Check sheet for the modelled part. Datum: model origin and axes. Units: mm. A direction names the side the tool comes from. Round coordinates to 2 decimals unless told otherwise and drop trailing zeros. Loops run counter-clockwise (first coordinate to the right, second up) from the corner with the lowest first, then second, coordinate; pieces in that order, holes last. Notation, with made-up numbers: (-32, 17.25) -> (7, 17.25) arc R25 cw to (7, 54.25) -> close; hole circle Ø1 at (75, 31.5). An arc over 180 degrees is marked (long way). One line per item, written item: value. Start each with the question number.
1. Cross-section at C-C on x = 89.5. Record the cut outline in (y, z), then the cut area to 3 significant figures.
2. Set-up check for faces 1 (the face through (29, 62, -7)), 2 (the face through (112, -60, -6)), 3 (the face through (33, 66, -7)), 4 (the face through (115, 62, -7)), 5 (the face through (-61.6, -51.1, 2.5)): record each of +Z, -Z, +X, -X, +Y, -Y from which the full face is reachable in a straight line by a thin tool's end or side.
3. Release check for a two-part mould opening along Y. For faces 6 (the face through (109, -63, -6)), 7 (the face through (31, 2, 5)), 8 (the face through (32.14, 84.86, 2.54)), 9 (the face through (127.15, -101.99, 2.46)) record: +Y half, -Y half, draft (parallel to the pull), parting line (faces both ways), or undercut.
4. Cross-section at B-B on y = 4.5. Record the cut outline in (x, z).
5. Cross-section at A-A on z = -12. Record the cut outline in (x, y).
6. Go/stop test with flat-tipped pins: pin 1 (3 mm diameter, centred on x = 49.5, y = 63.5, fed in from +Z); pin 2 (4 mm diameter, centred on x = 34.5, z = -7, fed in from +Y); pin 3 (1.5 mm diameter, centred on x = -101.5, z = 2.5, fed in from +Y); pin 4 (3.5 mm diameter, centred on x = -16.85, y = 58.25, fed in from -Z). Record where each tip stops, or that it passes through.
7. Material ranges on L1, parallel to Y at x = 79.5, z = 3.75; L2, parallel to X at y = 58.25, z = 2.45; L3, parallel to Y at x = -34.85, z = 2, recorded low to high.
from build123d import *

# Parameters (mm, degrees)
EXTRUDE_1_DEPTH       = 5
CUT_EXTRUDE_1_DEPTH   = 185.623942109
CUT_EXTRUDE_2_DEPTH   = 185.623942109
EXTRUDE_2_DEPTH       = 15
CUT_EXTRUDE_3_DEPTH   = 10
CUT_EXTRUDE_4_DEPTH   = 10
MIRROR_2_COPY_1_DEPTH = 15
MIRROR_2_COPY_2_DEPTH = 10
MIRROR_2_COPY_3_DEPTH = 10
SKETCH_7_R            = 1.6
CUT_EXTRUDE_5_DEPTH   = 186.16479147
SKETCH_8_R            = 1.6
CUT_EXTRUDE_6_DEPTH   = 186.16479147


with BuildPart() as part:
    # 草图1 → 凸台-拉伸1 (new body)
    with BuildSketch(Plane.XY):
        with BuildLine():
            Line((-51, 115), (-51, 121))
            ThreePointArc((-51, 121), (-48.071067812, 128.071067812), (-41, 131))
            Line((-41, 131), (29, 131))
            ThreePointArc((29, 131), (36.071067812, 128.071067812), (39, 121))
            Line((39, 121), (39, 115))
            ThreePointArc((39, 115), (41.928932188, 107.928932188), (49, 105))
            Line((49, 105), (120, 105))
            ThreePointArc((120, 105), (127.071067812, 102.071067812), (130, 95))
            Line((130, 95), (130, -95))
            ThreePointArc((130, -95), (127.071067812, -102.071067812), (120, -105))
            Line((120, -105), (49, -105))
            ThreePointArc((49, -105), (41.928932188, -107.928932188), (39, -115))
            Line((39, -115), (39, -121))
            ThreePointArc((39, -121), (36.071067812, -128.071067812), (29, -131))
            Line((29, -131), (-41, -131))
            ThreePointArc((-41, -131), (-48.071067812, -128.071067812), (-51, -121))
            Line((-51, -121), (-51, -115))
            ThreePointArc((-51, -115), (-53.928932188, -107.928932188), (-61, -105))
            Line((-61, -105), (-120, -105))
            ThreePointArc((-120, -105), (-127.071067812, -102.071067812), (-130, -95))
            Line((-130, -95), (-130, 95))
            ThreePointArc((-130, 95), (-127.071067812, 102.071067812), (-120, 105))
            Line((-120, 105), (-61, 105))
            ThreePointArc((-61, 105), (-53.928932188, 107.928932188), (-51, 115))
        make_face()
    extrude(amount=EXTRUDE_1_DEPTH)

    # 草图2 → 切除-拉伸1 (cut, through all)
    with BuildSketch(Plane.XY.offset(5)):
        with BuildLine():
            Line((10.846153846, -93.730769231), (52.846153846, -76.230769231))
            ThreePointArc((52.846153846, -76.230769231), (55.664100589, -76.503849117), (57, -79))
            Line((57, -79), (57, -96.5))
            ThreePointArc((57, -96.5), (56.121320344, -98.621320344), (54, -99.5))
            Line((54, -99.5), (12, -99.5))
            ThreePointArc((12, -99.5), (9.058257973, -97.088348405), (10.846153846, -93.730769231))
        make_face()
        Polygon((-108, 99.5), (-86, 99.5), (-82, 95.5), (-82, 73.5), (-86, 69.5), (-108, 69.5), (-112, 73.5), (-112, 95.5), align=None)
        Polygon((-108, -67), (-86, -67), (-82, -71), (-82, -93), (-86, -97), (-108, -97), (-112, -93), (-112, -71), align=None)
        Polygon((86, 97), (108, 97), (112, 93), (112, 76), (108, 72), (86, 72), (82, 76), (82, 93), align=None)
        Polygon((86, -69.5), (108, -69.5), (112, -73.5), (112, -90.5), (108, -94.5), (86, -94.5), (82, -90.5), (82, -73.5), align=None)
        with BuildLine():
            Line((12, 99.5), (54, 99.5))
            ThreePointArc((54, 99.5), (56.121320344, 98.621320344), (57, 96.5))
            Line((57, 96.5), (57, 79))
            ThreePointArc((57, 79), (55.664100589, 76.503849117), (52.846153846, 76.230769231))
            Line((52.846153846, 76.230769231), (10.846153846, 93.730769231))
            ThreePointArc((10.846153846, 93.730769231), (9.058257973, 97.088348405), (12, 99.5))
        make_face()
    extrude(amount=-CUT_EXTRUDE_1_DEPTH, mode=Mode.SUBTRACT)

    # 草图3 → 切除-拉伸2 (cut, through all)
    with BuildSketch(Plane(origin=(0, 0, 0), x_dir=(-1, 0, 0), z_dir=(0, 0, -1))):
        Polygon((57.7, 55), (-18, 55), (-26, 47), (-26, -47), (-18, -55), (57.7, -55), (65.7, -47), (65.7, 47), align=None)
    extrude(amount=-CUT_EXTRUDE_2_DEPTH, mode=Mode.SUBTRACT)

    # 草图4 → 凸台-拉伸2 (add)
    with BuildSketch(Plane(origin=(0, 0, 0), x_dir=(-1, 0, 0), z_dir=(0, 0, -1))):
        Polygon((-29, -55), (-29, -66), (-40, -66), (-40, -63), (-32, -63), (-32, -55), align=None)
    extrude_2 = extrude(amount=EXTRUDE_2_DEPTH)

    # 草图5 → 切除-拉伸3 (cut)
    with BuildSketch(Plane.XZ.offset(66)):
        Polygon((40, -5), (34.5, -15), (40, -15), align=None)
    cut_extrude_3 = extrude(amount=-CUT_EXTRUDE_3_DEPTH, mode=Mode.SUBTRACT)

    # 草图6 → 切除-拉伸4 (cut)
    with BuildSketch(Plane.ZY.offset(-29)):
        Polygon((-15, -60.5), (-5, -55), (-15, -55), align=None)
    cut_extrude_4 = extrude(amount=-CUT_EXTRUDE_4_DEPTH, mode=Mode.SUBTRACT)

    # 镜向1: 凸台-拉伸2, 切除-拉伸3, 切除-拉伸4 across plane
    add(extrude_2.mirror(Plane.ZY.offset(-72)))
    add(cut_extrude_3.mirror(Plane.ZY.offset(-72)), mode=Mode.SUBTRACT)
    add(cut_extrude_4.mirror(Plane.ZY.offset(-72)), mode=Mode.SUBTRACT)

    # 镜向2: 凸台-拉伸2, 切除-拉伸3, 切除-拉伸4 across plane
    add(extrude_2.mirror(Plane.ZX))
    add(cut_extrude_3.mirror(Plane.ZX), mode=Mode.SUBTRACT)
    add(cut_extrude_4.mirror(Plane.ZX), mode=Mode.SUBTRACT)

    # 镜向2 copy 1 sketch → 镜向2 copy 1 (add)
    with BuildSketch(Plane(origin=(144, 0, 0), x_dir=(1, 0, 0), z_dir=(0, 0, -1))):
        Polygon((-29, -55), (-29, -66), (-40, -66), (-40, -63), (-32, -63), (-32, -55), align=None)
    extrude(amount=MIRROR_2_COPY_1_DEPTH)

    # 镜向2 copy 2 sketch → 镜向2 copy 2 (cut)
    with BuildSketch(Plane(origin=(144, 66, 0), x_dir=(-1, 0, 0), z_dir=(0, 1, 0))):
        Polygon((40, -5), (34.5, -15), (40, -15), align=None)
    extrude(amount=-MIRROR_2_COPY_2_DEPTH, mode=Mode.SUBTRACT)

    # 镜向2 copy 3 sketch → 镜向2 copy 3 (cut)
    with BuildSketch(Plane(origin=(115, 0, 0), x_dir=(0, 0, 1), z_dir=(1, 0, 0))):
        Polygon((-15, -60.5), (-5, -55), (-15, -55), align=None)
    extrude(amount=-MIRROR_2_COPY_3_DEPTH, mode=Mode.SUBTRACT)

    # 草图7 → 切除-拉伸5 (cut, through all)
    with BuildSketch(Plane(origin=(0, 0, 0), x_dir=(-1, 0, 0), z_dir=(0, 0, -1))):
        with Locations((16.85, -58.25)):
            Circle(SKETCH_7_R)
        with Locations((22.85, -58.25)):
            Circle(SKETCH_7_R)
        with Locations((40.85, -58.25)):
            Circle(SKETCH_7_R)
        with Locations((34.85, -58.25)):
            Circle(SKETCH_7_R)
    cut_extrude_5 = extrude(amount=-CUT_EXTRUDE_5_DEPTH, mode=Mode.SUBTRACT)

    # 镜向3: 切除-拉伸5 across plane
    add(cut_extrude_5.mirror(Plane.ZX), mode=Mode.SUBTRACT)

    # 草图8 → 切除-拉伸6 (cut, through all)
    with BuildSketch(Plane(origin=(0, 0, 0), x_dir=(-1, 0, 0), z_dir=(0, 0, -1))):
        with Locations((-49.5, -63.495385915)):
            Circle(SKETCH_8_R)
        with Locations((-64.5, -63.495385915)):
            Circle(SKETCH_8_R)
        with Locations((-79.5, -63.495385915)):
            Circle(SKETCH_8_R)
        with Locations((-94.5, -63.495385915)):
            Circle(SKETCH_8_R)
    cut_extrude_6 = extrude(amount=-CUT_EXTRUDE_6_DEPTH, mode=Mode.SUBTRACT)

    # 镜向4: 切除-拉伸6 across plane
    add(cut_extrude_6.mirror(Plane.ZX), mode=Mode.SUBTRACT)


solid = part.part
Taken from the geometry:
1. outline: (-105, 0) -> (-94.5, 0) -> (-94.5, 5) -> (-105, 5) -> close; (-69.5, 0) -> (72, 0) -> (72, 5) -> (-69.5, 5) -> close; (97, 0) -> (105, 0) -> (105, 5) -> (97, 5) -> close
1. area: 800 mm2
2. face 1: -Z, -X, +Y, -Y
2. face 2: -Z
2. face 3: -Z, +X, -X, +Y
2. face 4: -Z, +X, +Y, -Y
2. face 5: +Z, -Z
3. face 6: undercut
3. face 7: draft
3. face 8: undercut
3. face 9: -Y half
4. outline: (-130, 0) -> (-65.7, 0) -> (-65.7, 5) -> (-130, 5) -> close; (26, 0) -> (130, 0) -> (130, 5) -> (26, 5) -> close
5. outline: (29, -66) -> (36.15, -66) -> (36.15, -63) -> (32, -63) -> (32, -58.85) -> (29, -58.85) -> close; (29, 58.85) -> (32, 58.85) -> (32, 63) -> (36.15, 63) -> (36.15, 66) -> (29, 66) -> close; (107.85, -66) -> (115, -66) -> (115, -58.85) -> (112, -58.85) -> (112, -63) -> (107.85, -63) -> close; (107.85, 63) -> (112, 63) -> (112, 58.85) -> (115, 58.85) -> (115, 66) -> (107.85, 66) -> close
6. pin 1: passes through
6. pin 2: stops at y = 66
6. pin 3: stops at y = 105
6. pin 4: stops at z = 0
7. L1: y = -105 to -65.1, -61.9 to 61.9, 65.1 to 105
7. L2: x = -130 to -42.45, -39.25 to -36.45, -33.25 to -24.45, -21.25 to -18.45, -15.25 to 130
7. L3: y = -131 to -59.85, -56.65 to -55, 55 to 56.65, 59.85 to 131
